Verification items for the finished model (mm, model axes). Face numbers are marked on the shaded views. A direction names the side the tool comes from. Round coordinates to 2 decimals unless told otherwise and drop trailing zeros. Loops run counter-clockwise (first coordinate to the right, second up) from the corner with the lowest first, then second, coordinate; pieces in that order, holes last. Notation, with made-up numbers: (-3, -19) -> (18, -19) arc R10 ccw to (18, -2) -> close; hole circle Ø3 at (-33, 23.25). An arc over 180 degrees is marked (long way). Use a Markdown table: item, result. Add a question column.
```python
from build123d import *

# Parameters (mm, degrees)
PAD061_DEPTH      = 1.4
PAD061_DEPTH_BACK = 1.4
SKETCH083_R       = 2.5
SKETCH083_R_2     = 1.5
POCKET035_DEPTH   = 7
FILLET036_R       = 1


with BuildPart() as part:
    # Sketch082 → Pad061 (new body, two sides)
    with BuildSketch(Plane.XY) as pad061_sk:
        with BuildLine():
            ThreePointArc((1.25, 5.170844), (0, 7.5), (-1.25, 5.170844))
            ThreePointArc((-1, 4.341688), (-1.063859, 4.7747), (-1.25, 5.170844))
            Line((-1, 4.341688), (-1, 1))
            Line((-1, 1), (-3.5, 1))
            Line((-3.5, 1), (-3.5, -1))
            Line((-3.5, -1), (3.5, -1))
            Line((3.5, -1), (3.5, 1))
            Line((3.5, 1), (1, 1))
            Line((1, 1), (1, 4.341688))
            ThreePointArc((1.25, 5.170844), (1.063859, 4.7747), (1, 4.341688))
        make_face()
    extrude(amount=-PAD061_DEPTH)
    extrude(pad061_sk.sketch, amount=PAD061_DEPTH_BACK)

    # Sketch083 (on Face4 of Pad061) → Pocket035 (cut)
    with BuildSketch(Plane(origin=(0, 1, 0), x_dir=(-1, 0, 0), z_dir=(0, 1, 0))):
        Circle(SKETCH083_R)
        Circle(SKETCH083_R_2, mode=Mode.SUBTRACT)
    extrude(amount=POCKET035_DEPTH, mode=Mode.SUBTRACT)

    # Fillet036
    fillet036_edges = [part.edges().sort_by_distance(p)[0] for p in [
        (-3.5, 0, -1.4),
        (-3.5, 0, 1.4),
        (3.5, 0, 1.4),
        (3.5, 0, -1.4),
    ]]
    fillet(fillet036_edges, radius=FILLET036_R)


solid = part.part
```
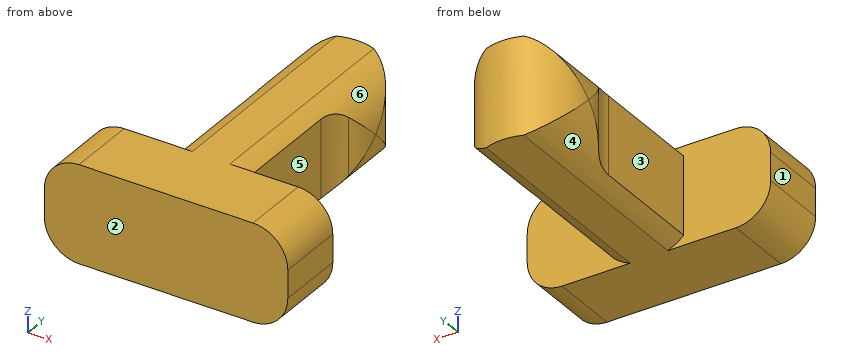
1) Sectioned sample at B-B on z = 0.2. Enter the section's corners in (x, y), then the cut area to 3 significant figures.
2) Sectioned sample at A-A on y = 3.75. Enter the section's corners in (x, z), then the cut area to 3 significant figures.
3) Thickness scan on line 1 (Y direction, x = -2.5, z = 0.7); line 2 (Z direction, x = -1, y = 5). Record the ranges inside material, lowest first.
4) Release check for a two-part mould opening along Y. For the marked faces 1, 2 and 3 record: released by +Y, released by -Y, zero draft, split by the parting line, or undercut.
5) Go/stop test with flat-tipped pins: pin 1 (1.4 mm diameter, centred on x = 2.5, z = -0.5, fed in from +Y); pin 2 (1 mm diameter, centred on y = 3.5, z = 0.5, fed in from -X). Record where each tip stops, or that it passes through.
6) Sectioned sample at C-C on x = 1.75. Enter the section's corners in (y, z), then the cut area to 3 significant figures.
7) Access from +Z, -Z, +X, -X, +Y, -Y to the whole of each face (thin tool, end or side, straight path). Record for the marked faces 4, 5 and 6.
8) Sectioned sample at D-D on y = 0.5. Enter the section's corners in (x, z).
Geometry results:
| question | item | result |
|---|---|---|
| 1 | outline | (-3.5, -1) -> (3.5, -1) -> (3.5, 1) -> (1, 1) -> (1, 4.34) arc R1.5 cw to (1.25, 5.17) arc R1.5 ccw to (1.49, 5.8) -> (1.49, 6.2) arc R1.5 ccw to (-1.49, 6.2) -> (-1.49, 5.8) arc R1.5 ccw to (-1.25, 5.17) arc R1.5 cw to (-1, 4.34) -> (-1, 1) -> (-3.5, 1) -> close |
| 1 | area | 28.4 mm^2 |
| 2 | outline | (-1, -1.12) arc R1.5 ccw to (-0.54, -1.4) -> (0.54, -1.4) arc R1.5 ccw to (1, -1.12) -> (1, 1.12) arc R1.5 ccw to (0.54, 1.4) -> (-0.54, 1.4) arc R1.5 ccw to (-1, 1.12) -> close |
| 2 | area | 5.38 mm^2 |
| 3 | line 1 | -1 to 1 |
| 3 | line 2 | -1.12 to 1.12 |
| 4 | face 1 | zero draft |
| 4 | face 2 | released by -Y |
| 4 | face 3 | undercut |
| 5 | pin 1 | y = 1 |
| 5 | pin 2 | x = -1 |
| 6 | outline | (-1, -1.4) -> (1, -1.4) -> (1, 1.4) -> (-1, 1.4) -> close |
| 6 | area | 5.60 mm^2 |
| 7 | face 4 | -Z, -X, +Y |
| 7 | face 5 | +Z, -Z, +X |
| 7 | face 6 | +Z, +X, +Y |
| 8 | outline | (-3.5, -0.4) arc R1 ccw to (-2.5, -1.4) -> (2.5, -1.4) arc R1 ccw to (3.5, -0.4) -> (3.5, 0.4) arc R1 ccw to (2.5, 1.4) -> (-2.5, 1.4) arc R1 ccw to (-3.5, 0.4) -> close |
